Solid Edge part; units mm, degrees
sketch "Sketch1" plane through (0, 0, 0) normal (0, 0, 1) x (1, 0, 0)
  circle A0 centre (0, 0) radius 25
extrude "Protrusion1" add sketch "Sketch1" against normal blind 5
sketch "Sketch2" plane through (0, 0, -5) normal (0, 0, -1) x (0, 1, 0)
  circle A0 centre (12.7279, 12.7279) radius 5
extrude "Legs_of_Table_Protrusion" add sketch "Sketch2" along normal blind 15
pattern_circular "Pattern1" count 4 over 360 about axis through (0, 0, 0) along (0, 0, 1) of "Legs_of_Table_Protrusion"
sketch "Sketch3" plane through (0, 0, -15) normal (0, 0, 1) x (1, 0, 0)
  line L0 (31.5442, 0) -> (39.5442, 0)
  arc A0 (22.3051, 22.3051) -> (31.5442, 0) centre (0, 0) cw
  line L1 (22.3051, 22.3051) -> (27.962, 27.962)
  arc A1 (27.962, 27.962) -> (39.5442, 0) centre (0, 0) cw
extrude "Seat_Protrusion" add sketch "Sketch3" along normal blind 5
sketch "Sketch4" plane through (30.9246, 13.981, -15) normal (0, 0, -1) x (0.7071, 0.7071, 0)
  circle A0 centre (-3.7911, 10.3241) radius 2.5
extrude "Protrusion2" add sketch "Sketch4" along normal up to vertex (5 mm away)
sketch "Sketch5" plane through (30.9246, 13.981, -15) normal (0, 0, -1) x (0.7071, 0.7071, 0)
  circle A0 centre (3.7911, -7.981) radius 2.5
extrude "Protrusion3" add sketch "Sketch5" along normal up to vertex (5 mm away)
pattern_circular "Pattern3" count 5 over 360 about axis through (0, 0, 0) along (0, 0, -1) of "Seat_Protrusion", "Protrusion2", "Protrusion3"
sketch "Sketch6" plane through (0, 0, 0) normal (0, 0, 1) x (1, 0, 0)
  line L0 (7.5, -7.5) -> (7.5, 7.5)
  line L1 (7.5, 7.5) -> (-7.5, 7.5)
  line L2 (-7.5, 7.5) -> (-7.5, -7.5)
  line L3 (-7.5, -7.5) -> (7.5, -7.5)
extrude "Button_Base_1" add sketch "Sketch6" along normal blind 2
sketch "Sketch7" plane through (0, 0, 2) normal (0, 0, 1) x (1, 0, 0)
  line L0 (-6.5, 6.5) -> (-6.5, -6.5)
  line L1 (-6.5, -6.5) -> (6.5, -6.5)
  line L2 (6.5, -6.5) -> (6.5, 6.5)
  line L3 (6.5, 6.5) -> (-6.5, 6.5)
  line L4 (-5, 5) -> (-5, -5)
  line L5 (-5, -5) -> (5, -5)
  line L6 (5, -5) -> (5, 5)
  line L7 (5, 5) -> (-5, 5)
extrude "Button_Base_2" add sketch "Sketch7" along normal blind 3
sketch "Sketch8" plane through (0, 0, 2) normal (0, 0, 1) x (0, -1, 0)
  circle A0 centre (0, 0) radius 4
extrude "Emergency_Button_Protrusion" add sketch "Sketch8" along normal blind 4
sketch "Sketch9" plane through (-35.7323, -1.6096, -20) normal (0, 0, -1) x (0, -1, 0)
  circle A0 centre (-1.6096, -35.7323) radius 40
extrude "Base_Protrusion" add sketch "Sketch9" along normal blind 2
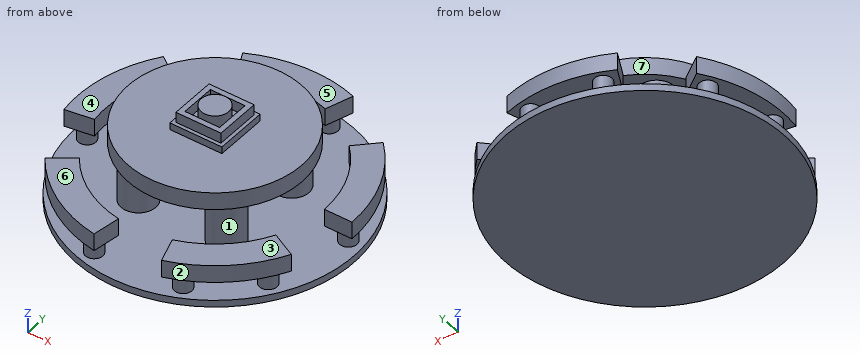
Can you work these out from the model? Positions are in its coordinate system, mm. Face numbers are marked on the shaded views. A direction names the side the tool comes from. Round coordinates to 2 decimals unless told otherwise and drop trailing zeros. Loops run counter-clockwise (first coordinate to the right, second up) from the corner with the lowest first, then second, coordinate; pieces in that order, holes last. Notation, with made-up numbers: (-22.5, -23) -> (23.5, -23) arc R15 ccw to (23.5, -6) -> close; hole circle Ø11 at (-9, -40). An arc over 180 degrees is marked (long way). One line per item, written item: value. Start each with the question number.
1. For the marked faces 4, 5, 6 and 7, which set-ups out of +Z, -Z, +X, -X, +Y, -Y let a thin tool reach every point of the face, with its end or its side?
2. If we section it at B-B, the plane z = 3.75: Write out the boundary of the cut face in (x, y).
3. If we section it at C-C, the plane z = -13: Give the number of separate pieces and of enclosed holes in the cut face, then the cut area to 3 significant figures.
4. For pin 1 (1 mm diameter, centred on x = -2.5, z = 1, fed in from +Y); pin 2 (0.9 mm diameter, centred on y = 1.5, z = 3, fed in from +X); pin 3 (4 mm diameter, centred on y = -6, z = -1.5, fed in from -X), each with a flat end and sliding along its axis, tell me the tip position at first contact or that it passes through.
5. If we section it at A-A, the plane x = 0: Write out the boundary of the cut face in (y, z), then the cut area to 3 significant figures.
6. If we mould it in two halves opening along Y, with no side actions, what happens to the marked faces 1, 2 and 3? For each: pulls with the +Y half, pulls with the -Y half, needs draft (parallel to the pull), parting line crosses it, or undercut.
7. If I drill on probe 1 along Z at (x, y) = (-9, 3.5); probe 2 along Y at (x, z) = (-11.5, -12.75); probe 3 along Z at (x, y) = (28, -21), over which ranges is the centre line in solid material (lowest first)?
Calculated:
1. face 4: +Z, -X, +Y, -Y
1. face 5: +Z, +X, -X, +Y
1. face 6: +Z, +X, -X, -Y
1. face 7: +Z
2. outline: (-6.5, -6.5) -> (6.5, -6.5) -> (6.5, 6.5) -> (-6.5, 6.5) -> close; circle Ø8 at (0, 0); hole (-5, -5) -> (5, -5) -> (5, 5) -> (-5, 5) -> close
3. separate pieces: 9
3. enclosed holes: 0
3. area: 1,430 mm²
4. pin 1: stops at y = 7.5
4. pin 2: stops at x = 6.5
4. pin 3: stops at x = -24.68
5. outline: (-40, -22) -> (40, -22) -> (40, -20) -> (-40, -20) -> close; (-25, -5) -> (25, -5) -> (25, 0) -> (7.5, 0) -> (7.5, 2) -> (6.5, 2) -> (6.5, 5) -> (5, 5) -> (5, 2) -> (4, 2) -> (4, 6) -> (-4, 6) -> (-4, 2) -> (-5, 2) -> (-5, 5) -> (-6.5, 5) -> (-6.5, 2) -> (-7.5, 2) -> (-7.5, 0) -> (-25, 0) -> close; (31.54, -15) -> (39.54, -15) -> (39.54, -10) -> (31.54, -10) -> close
5. area: 521 mm²
6. face 1: undercut
6. face 2: pulls with the -Y half
6. face 3: needs draft
7. probe 1: z = -22 to -20, -5 to 0
7. probe 2: y = -37.84 to -29.37, -17.57 to -7.88, 7.88 to 17.57, 29.37 to 37.84
7. probe 3: z = -22 to -10
